Can you work these out from the model? Positions are in its coordinate system, mm. A direction names the side the tool comes from. Give positions to 0.01 mm unless a question says otherwise; leave off trailing zeros. Order: outer loops, then holes, each group sorted by start corner. A loop starts at its lowest first (then second) coordinate and runs counter-clockwise, first axis right, second up. Notation, with made-up numbers: (81.5, 45.25) - (102.5, 45.25) arc R19 cw to (102.5, 78.25) - close; hole circle Ø8 at (41.25, 33.25). An arc over 180 degrees is marked (long way). Return JSON: item names as keys, results as strings.
```python
from build123d import *

# Parameters (mm, degrees)
SKETCH_R        = 70
PAD_DEPTH       = 15
SKETCH001_R     = 50
PAD001_DEPTH    = 80
SKETCH002_R     = 38
POCKET_DEPTH    = 150
SKETCH003_R     = 5
POCKET001_DEPTH = 100
SKETCH004_W     = 113.045652
SKETCH004_H     = 208.901421
POCKET002_DEPTH = 150


with BuildPart() as part:
    # Sketch → Pad (new body)
    with BuildSketch(Plane.XY):
        Circle(SKETCH_R)
    extrude(amount=PAD_DEPTH)

    # Sketch001 → Pad001 (join)
    with BuildSketch(Plane.XY):
        Circle(SKETCH001_R)
    extrude(amount=PAD001_DEPTH)

    # Sketch002 (on Face6 of Pad001) → Pocket (cut)
    with BuildSketch(Plane.XY.offset(80)):
        Circle(SKETCH002_R)
    extrude(amount=-POCKET_DEPTH, mode=Mode.SUBTRACT)

    # Sketch003 (on Face3 of Pocket) → Pocket001 (cut)
    with BuildSketch(Plane.XY.offset(15)):
        with Locations((57.5, 0)):
            Circle(SKETCH003_R)
    extrude(amount=-POCKET001_DEPTH, mode=Mode.SUBTRACT)

    # Sketch004 (on DatumPlane) → Pocket002 (cut)
    with BuildSketch(Plane.XY.offset(80)):
        with Locations((-36.229188, 6.106403)):
            Rectangle(SKETCH004_W, SKETCH004_H)
    extrude(amount=-POCKET002_DEPTH, mode=Mode.SUBTRACT)


solid = part.part
```
1. Suppose I cut it at C-C (x = 30). List the corners of the cut face in (y, z) for me, plus the area to 3 significant figures.
Checks:
{"outline": "(-63.25, 0) - (-23.32, 0) - (-23.32, 80) - (-40, 80) - (-40, 15) - (-63.25, 15) - close; (23.32, 0) - (63.25, 0) - (63.25, 15) - (40, 15) - (40, 80) - (23.32, 80) - close", "area": "3,370 mm^2"}
2. If I drill on L1, parallel to Y at x = 57.5, z = 3; L2, parallel to Y at x = 26, z = 18; L3, parallel to Z at x = 53, y = 10, over which ranges is the centre line in solid material (lowest first)? Write a range as [from, to].
Checks:
{"L1": "[-39.92, -5], [5, 39.92]", "L2": "[-42.71, -27.71], [27.71, 42.71]", "L3": "[0, 15]"}
3. Suppose I cut it at A-A (y = 0). List the corners of the cut face in (x, z) for me.
Checks:
{"outline": "(38, 0) - (52.5, 0) - (52.5, 15) - (50, 15) - (50, 80) - (38, 80) - close; (62.5, 0) - (70, 0) - (70, 15) - (62.5, 15) - close"}
4. On a 3-axis mill with a long thin cutter (end or side, diameter ignored), from which of +Z, -Z, +X, -X, +Y, -Y can I reach the whole of each face in a straight line? I mean faces 4 (the face through (50.3, 0.9, 15)), 5 (the face through (52.505, 0.22, 7.605)). Say none if no direction works.
Checks:
{"face 4": "+Z, +X", "face 5": "+Z, -Z"}
5. For pin 1 Ø2 at (x, y) = (52.5, -12.5) entering from +Z; pin 2 Ø10 at (y, z) = (25, 57) entering from +X; pin 3 Ø6 at (x, z) = (42.5, 34) entering from -Y; pin 4 Ø8 at (x, y) = (57.5, 0) entering from -Z, each with a flat end and sliding along its axis, tell me the tip position at first contact or that it passes through.
Checks:
{"pin 1": "z = 15", "pin 2": "x = 45.83", "pin 3": "y = -30.66", "pin 4": "through"}
6. Suppose I cut it at B-B (x = 57.5). List the corners of the cut face in (y, z) for me, plus the area to 3 significant figures.
Checks:
{"outline": "(-39.92, 0) - (-5, 0) - (-5, 15) - (-39.92, 15) - close; (5, 0) - (39.92, 0) - (39.92, 15) - (5, 15) - close", "area": "1,050 mm^2"}
7. Suppose I cut it at D-D (y = -16). List the corners of the cut face in (x, z) for me, plus the area to 3 significant figures.
Checks:
{"outline": "(34.47, 0) - (68.15, 0) - (68.15, 15) - (47.37, 15) - (47.37, 80) - (34.47, 80) - close", "area": "1,340 mm^2"}
8. Thinking about a two-plate mould opening in Y: for faces 1 (the face through (49.993, -0.807, 47.045)), 2 (the face through (37.996, -0.536, 40.56)), 3 (the face through (38.2, 0.6, 80)), which applies, +Y half, -Y half, draft (parallel to the pull), parting line (faces both ways), or undercut?
Checks:
{"face 1": "parting line", "face 2": "undercut", "face 3": "draft"}
